Model file for the job. Use its own axes, mm. Coordinates: 2 decimals unless noted, no trailing zeros. Return JSON: item names as keys, results as strings. Group by question number.
1) Pull direction X, two halves, no side cores. Call faces 1 (the cylindrical face through (1.264, -101.867, -57.486)), 2 (the flat face through (-63, -44, 0)): +X half, -X half, draft (parallel to the pull), parting line (faces both ways), or undercut.
2) Flat gauge pins, fed straight in: pin 1 (4 mm diameter, centred on y = -59.5, z = -8.5, fed in from +X); pin 2 (2 mm diameter, centred on x = -47.5, y = 17.5, fed in from +Z); pin 3 (5 mm diameter, centred on x = 32.5, y = 11, fed in from -Z). Where does each tip first touch, or does it go through?
3) Probe line 1 (X direction, y = -111, z = -26); line 2 (Z direction, x = 0, y = -110.5); line 3 (X direction, y = -23, z = -32.5). List the from-to ranges inside material, lowest first.
from build123d import *

# Parameters (mm, degrees)
F1_ANGLE    = 180
F2_T1_DEPTH = 235
F2_T3_DEPTH = 235


# Not quite as in the source:
# - a fillet or chamfer that OpenCascade refuses, or shapes differently, is made with other operations: its cross-section is extruded or revolved along the edge and cut away or added


with BuildPart() as f1:
    # F0 (on Top) → F1 (revolve)
    with BuildSketch(Plane.XY):
        with BuildLine():
            Line((55, 76.2), (45, 76.2))
            add(Edge.make_bspline(
                [(45, 76.2), (46.4314513107, 65.4743240031), (49.4342728448, 42.9745780396), (58.2913617327, 2.5444927944), (60.7679740967, -26.0894301808), (58.7809439185, -60.3358085831), (53.5427275811, -75.7766382868), (56.3670048957, -80.6107385976), (57.5, -82.55)],
                knots=[0, 0, 0, 0, 0.1935302552, 0.4059773556, 0.5886953586, 0.7831392141, 0.9130035116, 1, 1, 1, 1], degree=3))
            Line((57.5, -82.55), (57.5, -120.65))
            Line((57.5, -120.65), (67.5, -120.65))
            add(Edge.make_bspline(
                [(55, 76.2), (56.4448487865, 65.4735496208), (59.4077958305, 42.9708360316), (68.3641601176, 2.5594432328), (70.5377050341, -26.12710406), (69.5737841588, -60.0998956005), (67.2249671963, -76.0618392071), (67.611979836, -82.6108206706), (67.4592693335, -102.3954969726), (67.5036900604, -114.5662351269), (67.5, -120.65)],
                knots=[0, 0, 0, 0, 0.1503921233, 0.3154845037, 0.4574744391, 0.6084055945, 0.7088837212, 0.7740964569, 0.8870482285, 1, 1, 1, 1], degree=3))
        make_face()
    revolve(axis=Axis((0, 0, 0), (0, 1, 0)), revolution_arc=F1_ANGLE)

    # F2: fillet of radius 45 on 2 edges, made by hand

    # F2_s2 → F2_t1 (cut)
    with BuildSketch(Plane.YZ.offset(-67.5)):
        with BuildLine():
            ThreePointArc((76.2, -45), (63.0198051534, -13.1801948466), (31.2, 0))
            Line((31.2, 0), (76.2, 0))
            Line((76.2, 0), (76.2, -45))
        make_face()
    extrude(amount=F2_T1_DEPTH, mode=Mode.SUBTRACT)

    # F2_s4 → F2_t3 (cut)
    with BuildSketch(Plane.YZ.offset(-167.5)):
        with BuildLine():
            ThreePointArc((76.2, -45), (63.0198051534, -13.1801948466), (31.2, 0))
            Line((31.2, 0), (76.2, 0))
            Line((76.2, 0), (76.2, -45))
        make_face()
    extrude(amount=F2_T3_DEPTH, mode=Mode.SUBTRACT)


solid = f1.part
Answers below:
{
 "1": {"face 1": "undercut", "face 2": "draft"},
 "2": {"pin 1": "stops at x = 68.88", "pin 2": "stops at z = -25.61", "pin 3": "stops at z = -59"},
 "3": {"line 1": "x = -62.29 to -51.29, 51.29 to 62.29", "line 2": "z = -67.49 to -57.5", "line 3": "x = -61.88 to -50.36, 50.36 to 61.88"}
}
